Can you work these out from the drawing? Everything is in mm from the part's minimum corner. Round coordinates to 2 decimals unless told otherwise and drop trailing zeros. Loops run counter-clockwise (first coordinate to the right, second up) from the corner with the lowest first, then second, coordinate; pieces in that order, holes last. Notation, with made-up numbers: (38, 23) -> (57, 23) arc R13 cw to (57, 47) -> close; hole circle Ø2 at (16.5, 38.25). An arc over 180 degrees is marked (long way). One line per item, written item: value.
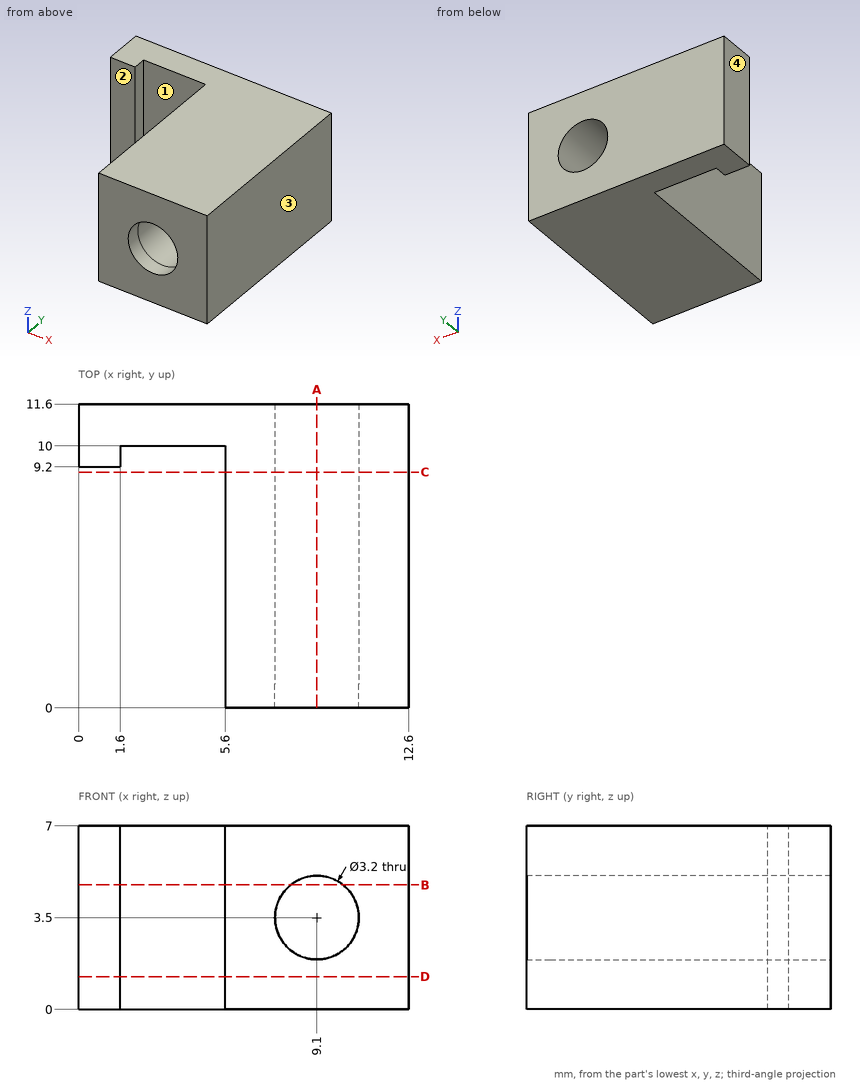
Item 1: I need wall thicknesses on line 1 (X direction, y = 5.25, z = 3.5); line 2 (Z direction, x = 9.1, y = 0.55); line 3 (X direction, y = 9.5, z = 1.25). Which ranges of each line are inside material? Lowest first, please. Write a range as from..to.
Output:
line 1: x = 5.6..7.5, 10.7..12.6
line 2: z = 0..1.9, 5.1..7
line 3: x = 0..1.6, 5.6..12.6
Item 2: If we section it at C-C on y = 9: List the corners of the cut face in (x, z) for me, plus the area to 3 significant figures.
Output:
outline: (5.6, 0) -> (12.6, 0) -> (12.6, 7) -> (5.6, 7) -> close; hole circle Ø3.2 at (9.1, 3.5)
area: 41.0 mm²
Item 3: If we section it at B-B on z = 4.75: List the corners of the cut face in (x, y) for me, plus the area to 3 significant figures.
Output:
outline: (0, 9.2) -> (1.6, 9.2) -> (1.6, 10) -> (5.6, 10) -> (5.6, 0) -> (8.1, 0) -> (8.1, 11.6) -> (0, 11.6) -> close; (10.1, 0) -> (12.6, 0) -> (12.6, 11.6) -> (10.1, 11.6) -> close
area: 68.3 mm²
Item 4: Will these pins go through, and if not, where does the flat tip stop? pin 1 Ø4 at (x, z) = (1.5, 5.5) entering from -Y; pin 2 Ø3 at (y, z) = (1, 6) entering from -X; pin 3 Ø2 at (x, y) = (5, 6.5) entering from +Z.
Output:
pin 1: stops at y = 9.2
pin 2: stops at x = 5.6
pin 3: stops at z = 7
Item 5: If we section it at A-A on x = 9.1: List the corners of the cut face in (y, z) for me.
Output:
outline: (0, 0) -> (11.6, 0) -> (11.6, 1.9) -> (0, 1.9) -> close; (0, 5.1) -> (11.6, 5.1) -> (11.6, 7) -> (0, 7) -> close
Item 6: If we mould it in two halves opening along X, with no side actions, what happens to the marked faces 1, 2, 3 and 4? For each: released by +X, released by -X, zero draft, split by the parting line, or undercut.
Output:
face 1: undercut
face 2: zero draft
face 3: released by +X
face 4: released by -X
Item 7: If we section it at D-D on z = 1.25: List the corners of the cut face in (x, y) for me, plus the area to 3 significant figures.
Output:
outline: (0, 9.2) -> (1.6, 9.2) -> (1.6, 10) -> (5.6, 10) -> (5.6, 0) -> (12.6, 0) -> (12.6, 11.6) -> (0, 11.6) -> close
area: 91.4 mm²
